```python
from build123d import *

# Parameters (mm, degrees)
F0_R     = 2.75
F1_DEPTH = 4


with BuildPart() as f1:
    # F0 (on Front) → F1 (new body)
    with BuildSketch(Plane.XZ):
        with BuildLine():
            add(Edge.make_bspline(
                [(-100, 95), (-81.2941622631, 94.4236036805), (-47.5910411734, 87.3203708431), (-25.3869639524, 88.2401502703), (-20.5, 88.75608063)],
                knots=[0, 0, 0, 0, 0.5689678783, 0.7432926029, 0.7432926029, 0.7432926029, 0.7432926029], degree=3))
            ThreePointArc((-100, 95), (-115, 80), (-100, 65))
            add(Edge.make_bspline(
                [(-100, 65), (-81.2941622631, 65.5763963195), (-47.5910411734, 72.6796291569), (-25.3869639524, 71.7598497297), (-20.5, 71.24391937)],
                knots=[0, 0, 0, 0, 0.5689678783, 0.7432926029, 0.7432926029, 0.7432926029, 0.7432926029], degree=3))
            add(Edge.make_bspline(
                [(-20.5, 71.24391937), (-19.6576755147, 71.1549928343), (-18.8248746074, 71.0571473907), (-18, 70.9511054936)],
                knots=[0.7432926029, 0.7432926029, 0.7432926029, 0.7432926029, 0.7733394757, 0.7733394757, 0.7733394757, 0.7733394757], degree=3))
            add(Edge.make_bspline(
                [(-18, 70.9511054936), (-11.7775051442, 70.1511715966), (-6.006059288, 68.884815508), (0, 67.4621646617)],
                knots=[0.7733394757, 0.7733394757, 0.7733394757, 0.7733394757, 1, 1, 1, 1], degree=3))
            add(Edge.make_bspline(
                [(18, 70.9511054936), (11.7775051442, 70.1511715966), (6.006059288, 68.884815508), (0, 67.4621646617)],
                knots=[0.7733394757, 0.7733394757, 0.7733394757, 0.7733394757, 1, 1, 1, 1], degree=3))
            add(Edge.make_bspline(
                [(20.5, 71.24391937), (19.6576755147, 71.1549928343), (18.8248746074, 71.0571473907), (18, 70.9511054936)],
                knots=[0.7432926029, 0.7432926029, 0.7432926029, 0.7432926029, 0.7733394757, 0.7733394757, 0.7733394757, 0.7733394757], degree=3))
            add(Edge.make_bspline(
                [(100, 65), (81.2941622631, 65.5763963195), (47.5910411734, 72.6796291569), (25.3869639524, 71.7598497297), (20.5, 71.24391937)],
                knots=[0, 0, 0, 0, 0.5689678783, 0.7432926029, 0.7432926029, 0.7432926029, 0.7432926029], degree=3))
            ThreePointArc((100, 65), (115, 80), (100, 95))
            add(Edge.make_bspline(
                [(100, 95), (81.2941622631, 94.4236036805), (47.5910411734, 87.3203708431), (25.3869639524, 88.2401502703), (20.5, 88.75608063)],
                knots=[0, 0, 0, 0, 0.5689678783, 0.7432926029, 0.7432926029, 0.7432926029, 0.7432926029], degree=3))
            add(Edge.make_bspline(
                [(20.5, 88.75608063), (19.6576755147, 88.8450071657), (18.8248746074, 88.9428526093), (18, 89.0488945064)],
                knots=[0.7432926029, 0.7432926029, 0.7432926029, 0.7432926029, 0.7733394757, 0.7733394757, 0.7733394757, 0.7733394757], degree=3))
            add(Edge.make_bspline(
                [(18, 89.0488945064), (11.7775051442, 89.8488284034), (6.006059288, 91.115184492), (0, 92.5378353383)],
                knots=[0.7733394757, 0.7733394757, 0.7733394757, 0.7733394757, 1, 1, 1, 1], degree=3))
            add(Edge.make_bspline(
                [(-18, 89.0488945064), (-11.7775051442, 89.8488284034), (-6.006059288, 91.115184492), (0, 92.5378353383)],
                knots=[0.7733394757, 0.7733394757, 0.7733394757, 0.7733394757, 1, 1, 1, 1], degree=3))
            add(Edge.make_bspline(
                [(-20.5, 88.75608063), (-19.6576755147, 88.8450071657), (-18.8248746074, 88.9428526093), (-18, 89.0488945064)],
                knots=[0.7432926029, 0.7432926029, 0.7432926029, 0.7432926029, 0.7733394757, 0.7733394757, 0.7733394757, 0.7733394757], degree=3))
        make_face()
        with BuildLine():
            Line((-98.4, 72), (-98.4, 70.5))
            ThreePointArc((-98.4, 70.5), (-100, 68.9), (-101.6, 70.5))
            Line((-101.6, 70.5), (-101.6, 72))
            ThreePointArc((-101.6, 72), (-100, 73.6), (-98.4, 72))
        make_face(mode=Mode.SUBTRACT)
        with BuildLine():
            ThreePointArc((-109.5, 78.4), (-111.1, 80), (-109.5, 81.6))
            Line((-109.5, 81.6), (-108, 81.6))
            ThreePointArc((-108, 81.6), (-106.4, 80), (-108, 78.4))
            Line((-108, 78.4), (-109.5, 78.4))
        make_face(mode=Mode.SUBTRACT)
        with Locations((-100, 80)):
            Circle(F0_R, mode=Mode.SUBTRACT)
        with BuildLine():
            Line((-90.5, 78.4), (-92, 78.4))
            ThreePointArc((-92, 78.4), (-93.6, 80), (-92, 81.6))
            Line((-92, 81.6), (-90.5, 81.6))
            ThreePointArc((-90.5, 81.6), (-88.9, 80), (-90.5, 78.4))
        make_face(mode=Mode.SUBTRACT)
        with BuildLine():
            Line((101.6, 72), (101.6, 70.5))
            ThreePointArc((101.6, 70.5), (100, 68.9), (98.4, 70.5))
            Line((98.4, 70.5), (98.4, 72))
            ThreePointArc((98.4, 72), (100, 73.6), (101.6, 72))
        make_face(mode=Mode.SUBTRACT)
        with BuildLine():
            ThreePointArc((90.5, 78.4), (88.9, 80), (90.5, 81.6))
            Line((90.5, 81.6), (92, 81.6))
            ThreePointArc((92, 81.6), (93.6, 80), (92, 78.4))
            Line((92, 78.4), (90.5, 78.4))
        make_face(mode=Mode.SUBTRACT)
        with Locations((100, 80)):
            Circle(F0_R, mode=Mode.SUBTRACT)
        with BuildLine():
            Line((109.5, 78.4), (108, 78.4))
            ThreePointArc((108, 78.4), (106.4, 80), (108, 81.6))
            Line((108, 81.6), (109.5, 81.6))
            ThreePointArc((109.5, 81.6), (111.1, 80), (109.5, 78.4))
        make_face(mode=Mode.SUBTRACT)
        with BuildLine():
            ThreePointArc((-101.6, 89.5), (-100, 91.1), (-98.4, 89.5))
            Line((-98.4, 89.5), (-98.4, 88))
            ThreePointArc((-98.4, 88), (-100, 86.4), (-101.6, 88))
            Line((-101.6, 88), (-101.6, 89.5))
        make_face(mode=Mode.SUBTRACT)
        with BuildLine():
            Line((98.4, 88), (98.4, 89.5))
            ThreePointArc((98.4, 89.5), (100, 91.1), (101.6, 89.5))
            Line((101.6, 89.5), (101.6, 88))
            ThreePointArc((101.6, 88), (100, 86.4), (98.4, 88))
        make_face(mode=Mode.SUBTRACT)
        with BuildLine():
            Line((-20.5, 95), (-20.5, 88.75608063))
            add(Edge.make_bspline(
                [(-20.5, 88.75608063), (-19.6576755147, 88.8450071657), (-18.8248746074, 88.9428526093), (-18, 89.0488945064)],
                knots=[0.7432926029, 0.7432926029, 0.7432926029, 0.7432926029, 0.7733394757, 0.7733394757, 0.7733394757, 0.7733394757], degree=3))
            Line((-18, 89.0488945064), (-18, 95))
            Line((-18, 95), (-20.5, 95))
        make_face()
        with BuildLine():
            add(Edge.make_bspline(
                [(-20.5, 71.24391937), (-19.6576755147, 71.1549928343), (-18.8248746074, 71.0571473907), (-18, 70.9511054936)],
                knots=[0.7432926029, 0.7432926029, 0.7432926029, 0.7432926029, 0.7733394757, 0.7733394757, 0.7733394757, 0.7733394757], degree=3))
            Line((-20.5, 71.24391937), (-20.5, 65))
            Line((-20.5, 65), (-18, 65))
            Line((-18, 65), (-18, 70.9511054936))
        make_face()
        with BuildLine():
            Line((-18, 95), (-18, 89.0488945064))
            add(Edge.make_bspline(
                [(-18, 89.0488945064), (-11.7775051442, 89.8488284034), (-6.006059288, 91.115184492), (0, 92.5378353383)],
                knots=[0.7733394757, 0.7733394757, 0.7733394757, 0.7733394757, 1, 1, 1, 1], degree=3))
            add(Edge.make_bspline(
                [(18, 89.0488945064), (11.7775051442, 89.8488284034), (6.006059288, 91.115184492), (0, 92.5378353383)],
                knots=[0.7733394757, 0.7733394757, 0.7733394757, 0.7733394757, 1, 1, 1, 1], degree=3))
            Line((18, 89.0488945064), (18, 95))
            Line((18, 95), (18, 97.7))
            Line((18, 97.7), (20.5, 97.7))
            Line((20.5, 97.7), (20.5, 100.4))
            Line((20.5, 100.4), (-20.5, 100.4))
            Line((-20.5, 100.4), (-20.5, 97.7))
            Line((-20.5, 97.7), (-18, 97.7))
            Line((-18, 97.7), (-18, 95))
        make_face()
        with BuildLine():
            add(Edge.make_bspline(
                [(-18, 70.9511054936), (-11.7775051442, 70.1511715966), (-6.006059288, 68.884815508), (0, 67.4621646617)],
                knots=[0.7733394757, 0.7733394757, 0.7733394757, 0.7733394757, 1, 1, 1, 1], degree=3))
            Line((-18, 70.9511054936), (-18, 65))
            Line((-18, 65), (-18, 62.3))
            Line((-18, 62.3), (-20.5, 62.3))
            Line((-20.5, 62.3), (-20.5, 59.6))
            Line((-20.5, 59.6), (20.5, 59.6))
            Line((20.5, 59.6), (20.5, 62.3))
            Line((20.5, 62.3), (18, 62.3))
            Line((18, 62.3), (18, 65))
            Line((18, 65), (18, 70.9511054936))
            add(Edge.make_bspline(
                [(18, 70.9511054936), (11.7775051442, 70.1511715966), (6.006059288, 68.884815508), (0, 67.4621646617)],
                knots=[0.7733394757, 0.7733394757, 0.7733394757, 0.7733394757, 1, 1, 1, 1], degree=3))
        make_face()
        with BuildLine():
            Line((18, 95), (18, 89.0488945064))
            add(Edge.make_bspline(
                [(20.5, 88.75608063), (19.6576755147, 88.8450071657), (18.8248746074, 88.9428526093), (18, 89.0488945064)],
                knots=[0.7432926029, 0.7432926029, 0.7432926029, 0.7432926029, 0.7733394757, 0.7733394757, 0.7733394757, 0.7733394757], degree=3))
            Line((20.5, 88.75608063), (20.5, 95))
            Line((20.5, 95), (18, 95))
        make_face()
        with BuildLine():
            add(Edge.make_bspline(
                [(20.5, 71.24391937), (19.6576755147, 71.1549928343), (18.8248746074, 71.0571473907), (18, 70.9511054936)],
                knots=[0.7432926029, 0.7432926029, 0.7432926029, 0.7432926029, 0.7733394757, 0.7733394757, 0.7733394757, 0.7733394757], degree=3))
            Line((18, 70.9511054936), (18, 65))
            Line((18, 65), (20.5, 65))
            Line((20.5, 65), (20.5, 71.24391937))
        make_face()
    extrude(amount=F1_DEPTH)


solid = f1.part
```
Can you work these out from the model? Positions are in its coordinate system, mm. A direction names the side the tool comes from. Coordinates: 2 decimals unless noted, no trailing zeros.
1. Thinking about a two-plate mould opening in X: for faces 1 (the face through (-20.5, -2, 68)), 2 (the face through (2, -4, 80)), 3 (the face through (-115, -2, 80)), 4 (the face through (-102.747, -1.972, 80.121)), which applies, +X half, -X half, draft (parallel to the pull), parting line (faces both ways), or undercut?
2. I need wall thicknesses on line 1 (Z direction, x = -100, y = -3); line 2 (Z direction, x = -102.5, y = -1.85); line 3 (Z direction, x = 99, y = -1.75). Which ranges of each line are inside material? Lowest first, please.
3. I'm going to push flat-ended pins straight in: pin 1 (1.2 mm diameter, centred on y = -2, z = 71, fed in from -X); pin 2 (1.4 mm diameter, centred on y = -1, z = 98.5, fed in from +X); pin 3 (1 mm diameter, centred on x = 28, y = -2, fed in from -Z). Where does each tip first touch, or does it pass through?
4. If we section it at A-A (y = -3.3): Give the number of separate pieces and of enclosed holes in the cut face, then the cut area to 3 significant figures.
5. For faces 5 (the face through (97.253, -1.972, 80.121)), 6 (the face through (20.5, -2, 92)), 7 (the face through (20.5, -2, 68)), which set-ups out of +Z, -Z, +X, -X, +Y, -Y let a thin tool reach every point of the face, with its end or its side?
Entries:
1. face 1: undercut
1. face 2: draft
1. face 3: -X half
1. face 4: undercut
2. line 1: z = 65 to 68.9, 73.6 to 77.25, 82.75 to 86.4, 91.1 to 95
2. line 2: z = 65.21 to 78.85, 81.15 to 94.79
2. line 3: z = 65.04 to 69.25, 73.25 to 77.44, 82.56 to 86.75, 90.75 to 94.96
3. pin 1: stops at x = -112.43
3. pin 2: stops at x = 20.5
3. pin 3: stops at z = 71.75
4. separate pieces: 1
4. enclosed holes: 10
4. area: 5,700 mm2
5. face 5: +Y, -Y
5. face 6: +Z, +Y, -Y
5. face 7: -Z, +Y, -Y
